from build123d import *

# Parameters (mm, degrees)
EXTRUDE1_DEPTH  = 60
SKETCH2_R       = 3
EXTRUDE2_DEPTH  = 3.5
SKETCH_R        = 1.75
EXTRUDE3_DEPTH  = 7
LPATTERN1_COUNT = 45
LPATTERN1_PITCH = 50


with BuildPart() as part:
    # Sketch1 → Extrude1 (new body)
    with BuildSketch(Plane.XY):
        with BuildLine():
            Line((-4.5, -3), (4.5, -3))
            Line((4.5, -3), (4.5, 0))
            ThreePointArc((4.5, 0), (3.93077967, 0.177814974), (3.563991137, 0.648023568))
            Line((3.563991137, 0.648023568), (3.235073025, 0.648023568))
            Line((3.235073025, 0.648023568), (3.235073025, 1.351976432))
            Line((3.235073025, 1.351976432), (3.563991137, 1.351976432))
            ThreePointArc((3.563991137, 1.351976432), (3.93077967, 1.822185026), (4.5, 2))
            Line((4.5, 2), (4.5, 3))
            Line((4.5, 3), (-4.5, 3))
            Line((-4.5, 3), (-4.5, 2))
            ThreePointArc((-4.5, 2), (-3.93077967, 1.822185026), (-3.563991137, 1.351976432))
            Line((-3.563991137, 1.351976432), (-3.235073025, 1.351976432))
            Line((-3.235073025, 1.351976432), (-3.235073025, 0.648023568))
            Line((-3.235073025, 0.648023568), (-3.563991137, 0.648023568))
            ThreePointArc((-3.563991137, 0.648023568), (-3.93077967, 0.177814974), (-4.5, 0))
            Line((-4.5, 0), (-4.5, -3))
        make_face()
    extrude(amount=EXTRUDE1_DEPTH)

    # Sketch2 → Extrude2 (cut)
    with BuildSketch(Plane(origin=(0, 3, 0), x_dir=(1, 0, 0), z_dir=(0, 1, 0))):
        with Locations((0, -5)):
            Circle(SKETCH2_R)
    extrude2 = extrude(amount=-EXTRUDE2_DEPTH, mode=Mode.SUBTRACT)

    # Sketch → Extrude3 (cut, through all)
    with BuildSketch(Plane(origin=(0, 3, 0), x_dir=(1, 0, 0), z_dir=(0, 1, 0))):
        with Locations((0, -5)):
            Circle(SKETCH_R)
    extrude3 = extrude(amount=-EXTRUDE3_DEPTH, mode=Mode.SUBTRACT)

    # LPattern1: Extrude2, Extrude3 ×45
    with Locations(*[(0, 0, i * LPATTERN1_PITCH) for i in range(1, LPATTERN1_COUNT)]):
        add(extrude2, mode=Mode.SUBTRACT)
        add(extrude3, mode=Mode.SUBTRACT)


solid = part.part
Source: CAD feature listing. Evaluate the final solid. Frame: model axes, mm. A direction names the side the tool comes from. Coordinates: 2 decimals unless noted, no trailing zeros. Order: outer loops, then holes, each group sorted by start corner. A loop starts at its lowest first (then second) coordinate and runs counter-clockwise, first axis right, second up.
Item 1: First-contact query: P1, Ø3, axis at x = 0, z = 5, coming from the -Y side; P2, Ø0.8, axis at y = 1, z = 40.5, coming from the +X side; P3, Ø1.8, axis at x = 1, z = 5.5, coming from the +Y side. Flat tips, straight axial feed; report the tip coordinate or a pass-through.
Output values:
P1: passes through
P2: stops at x = 3.58
P3: stops at y = -0.5
Item 2: Cut plane C-C (z = 27.5). Return loops of the section in (x, y), plus the area to 3 significant figures.
Output values:
outline: (-4.5, -3) - (4.5, -3) - (4.5, 0) arc R1 cw to (3.56, 0.65) - (3.24, 0.65) - (3.24, 1.35) - (3.56, 1.35) arc R1 cw to (4.5, 2) - (4.5, 3) - (-4.5, 3) - (-4.5, 2) arc R1 cw to (-3.56, 1.35) - (-3.24, 1.35) - (-3.24, 0.65) - (-3.56, 0.65) arc R1 cw to (-4.5, 0) - close
area: 50.5 mm2
Item 3: Material intervals for line 1 (Z direction, x = 0, y = 0.85); line 2 (Z direction, x = 0, y = -2.3); line 3 (Y direction, x = -3.5, z = 22.5), sorted ascending.
Output values:
line 1: z = 0 to 2, 8 to 52, 58 to 60
line 2: z = 0 to 3.25, 6.75 to 53.25, 56.75 to 60
line 3: y = -3 to 0.65, 1.35 to 3
Item 4: Cut plane B-B (y = -2.4). Return loops of the section in (x, z).
Output values:
outline: (-4.5, 0) - (4.5, 0) - (4.5, 60) - (-4.5, 60) - close; hole circle Ø3.5 at (0, 5); hole circle Ø3.5 at (0, 55)
Item 5: Cut plane D-D (z = 5). Return loops of the section in (x, y).
Output values:
outline: (-4.5, -3) - (-1.75, -3) - (-1.75, -0.5) - (-3, -0.5) - (-3, 3) - (-4.5, 3) - (-4.5, 2) arc R1 cw to (-3.56, 1.35) - (-3.24, 1.35) - (-3.24, 0.65) - (-3.56, 0.65) arc R1 cw to (-4.5, 0) - close; (1.75, -3) - (4.5, -3) - (4.5, 0) arc R1 cw to (3.56, 0.65) - (3.24, 0.65) - (3.24, 1.35) - (3.56, 1.35) arc R1 cw to (4.5, 2) - (4.5, 3) - (3, 3) - (3, -0.5) - (1.75, -0.5) - close
Item 6: Pull-direction query (X, two-part tool) for faces 6 (the face through (0, 1, 52)), 7 (the face through (4.5, 2.5, 29.6)), 8 (the face through (0, 0, 60)); classes: pulls with the +X half, pulls with the -X half, needs draft (parallel to the pull), parting line crosses it, or undercut.
Output values:
face 6: undercut
face 7: pulls with the +X half
face 8: needs draft
Item 7: Set-up query: faces 1 (the face through (0, -3, 30)), 2 (the face through (2, -0.5, 5)), 3 (the face through (-3.9, 0.2, 29.6)), 4 (the face through (0, 3, 30)), 5 (the face through (3.9, 1.8, 29.6)). Return all of +Z, -Z, +X, -X, +Y, -Y with unobstructed straight access to the full face (end or side cutting, diameter ignored); none if empty.
Output values:
face 1: +Z, -Z, +X, -X, -Y
face 2: +Y
face 3: +Z, -Z, -X
face 4: +Z, -Z, +X, -X, +Y
face 5: +Z, -Z, +X
Item 8: Cut plane A-A (x = 0). Return loops of the section in (y, z).
Output values:
outline: (-3, 0) - (3, 0) - (3, 2) - (-0.5, 2) - (-0.5, 3.25) - (-3, 3.25) - close; (-3, 6.75) - (-0.5, 6.75) - (-0.5, 8) - (3, 8) - (3, 52) - (-0.5, 52) - (-0.5, 53.25) - (-3, 53.25) - close; (-3, 56.75) - (-0.5, 56.75) - (-0.5, 58) - (3, 58) - (3, 60) - (-3, 60) - close
